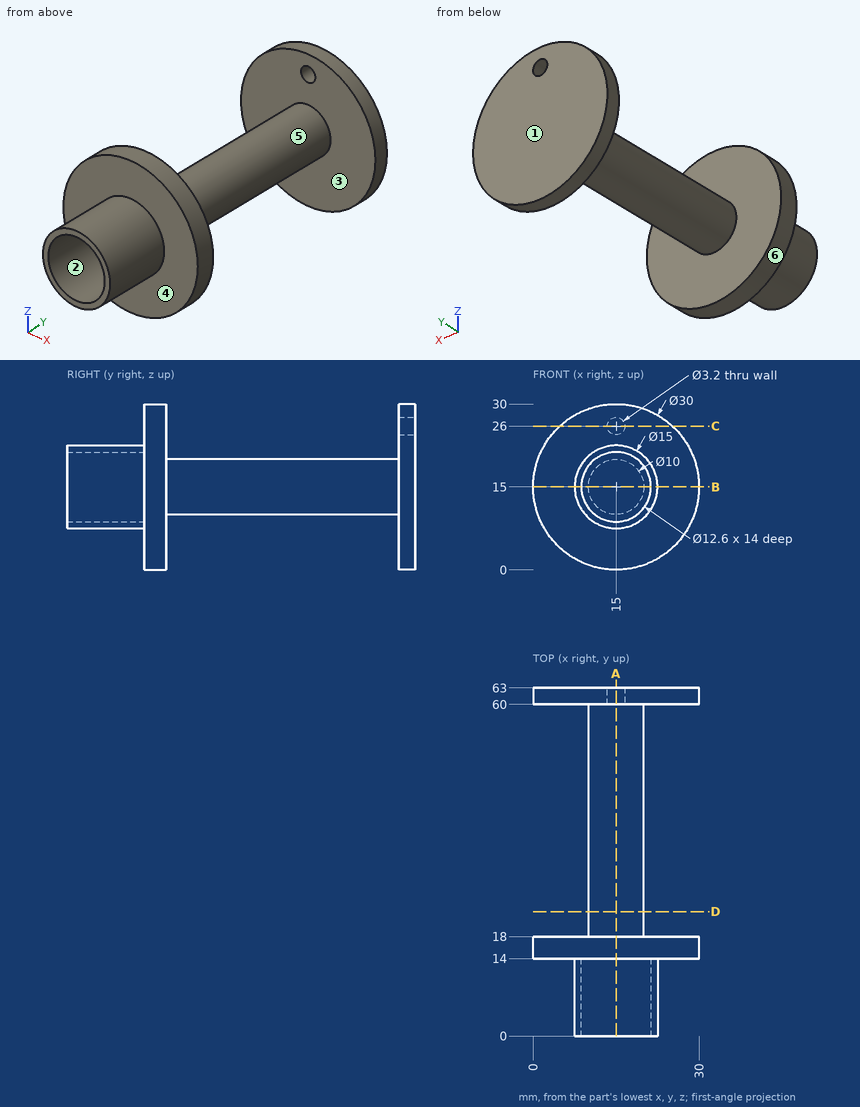
Here's the drawing with two shaded views (mm, measured from the low corner). I have some questions. A direction names the side the tool comes from. Coordinates: 2 decimals unless noted, no trailing zeros. Order: outer loops, then holes, each group sorted by start corner. A loop starts at its lowest first (then second) coordinate and runs counter-clockwise, first axis right, second up.
Q1. Suppose I cut it at D-D on y = 22.5. Please give me the cut outline in (x, z), and give its area (3 significant figures).
Q2. Thinking about a two-plate mould opening in Y: for the marked faces 1, 2 and 3, which applies, released by +Y, released by -Y, zero draft, split by the parting line, or undercut?
Q3. Suppose I cut it at C-C on z = 26. Please give me the cut outline in (x, y).
Q4. Suppose I cut it at B-B on z = 15. Please give me the cut outline in (x, y).
Q5. Suppose I cut it at A-A on x = 15. Please give me the cut outline in (y, z), and give its area (3 significant figures).
Q6. Please list where these lines run through material, in increasing order: L1, parallel to Y at x = 25.5, z = 6; L2, parallel to Z at x = 15, y = 60.85; L3, parallel to Y at x = 16.5, z = 21.25.
Q7. Which directions (+Z, -Z, +X, -X, +Y, -Y) give clear straight access to the entire face, cutting with the end or side of a thin tool? Please do the marked faces 4, 5 and 6.
Q8. Will these pins go through, and if not, where does the flat tip stop? pin 1 (2 mm diameter, centred on x = 21.5, y = 31.5, fed in from +Z); pin 2 (1.5 mm diameter, centred on x = 17.5, y = 28, fed in from +Z); pin 3 (6 mm diameter, centred on y = 34.5, z = 22, fed in from -X); pin 4 (3 mm diameter, centred on x = 15, z = 26, fed in from +Y).
Answer:
1. outline: circle Ø10 at (15, 15)
1. area: 78.5 mm2
2. face 1: released by +Y
2. face 2: zero draft
2. face 3: undercut
3. outline: (4.8, 14) - (25.2, 14) - (25.2, 18) - (4.8, 18) - close; (4.8, 60) - (13.4, 60) - (13.4, 63) - (4.8, 63) - close; (16.6, 60) - (25.2, 60) - (25.2, 63) - (16.6, 63) - close
4. outline: (0, 14) - (7.5, 14) - (7.5, 0) - (8.7, 0) - (8.7, 14) - (21.3, 14) - (21.3, 0) - (22.5, 0) - (22.5, 14) - (30, 14) - (30, 18) - (20, 18) - (20, 60) - (30, 60) - (30, 63) - (0, 63) - (0, 60) - (10, 60) - (10, 18) - (0, 18) - close
5. outline: (0, 7.5) - (14, 7.5) - (14, 0) - (18, 0) - (18, 10) - (60, 10) - (60, 0) - (63, 0) - (63, 24.4) - (60, 24.4) - (60, 20) - (18, 20) - (18, 30) - (14, 30) - (14, 22.5) - (0, 22.5) - (0, 21.3) - (14, 21.3) - (14, 8.7) - (0, 8.7) - close; (60, 27.6) - (63, 27.6) - (63, 30) - (60, 30) - close
5. area: 654 mm2
6. L1: y = 14 to 18, 60 to 63
6. L2: z = 0 to 24.4, 27.6 to 30
6. L3: y = 0 to 18, 60 to 63
7. face 4: -Y
7. face 5: none
7. face 6: +Y, -Y
8. pin 1: passes through
8. pin 2: stops at z = 19.68
8. pin 3: stops at x = 12
8. pin 4: stops at y = 18
